Read the model definition and answer for the solid it produces. Units are mm, in the model's axes. A direction names the side the tool comes from. Coordinates: 2 decimals unless noted, no trailing zeros. Write each loop counter-clockwise with the first axis right and the second up, starting at its lowest first coordinate (ties: lowest second). Pieces come first, ordered by that corner, then holes. Notation, with made-up numbers: (11, 13) -> (48, 13) arc R35 ccw to (48, 51) -> close; hole circle Ø11 at (6, 52.25). An arc over 180 degrees is marked (long way). Answer in a Markdown table with one row per item. Add a question column.
Item 1: Section C-C on y = -12 is taken. Write down the section's boundary in (x, z), then the cut area to 3 significant figures.
Item 2: Section D-D on z = -22.5 is taken. Write down the section's boundary in (x, y).
Item 3: Given pin 1 Ø2.5 at (y, z) = (0, 22.5) entering from -X; pin 2 Ø2 at (x, y) = (-5, -8) entering from -Z; pin 3 Ø2 at (x, y) = (-5.5, -0.5) entering from +Z; pin 4 Ø4 at (y, z) = (2.5, 8) entering from -X, each flat-ended and moving along its own axis, determine where each tip first touches the part or whether it passes through.
Item 4: Section A-A on x = -2 is taken. Write down the section's boundary in (y, z), then the cut area to 3 significant figures.
Item 5: For a pull along X with two mould halves and no side action, classify faces 1 (the face through (4.3, 1.26, -16.62)), 2 (the face through (-3, -9, -12)), 3 (the face through (-4.285, 3.177, -8.031)), 4 (the face through (-5, -7, -8.332)) as +X half, -X half, draft (parallel to the pull), parting line (faces both ways), or undercut.
Item 6: Section B-B on y = -4.5 is taken. Write down the section's boundary in (x, z).
Item 7: Which of the six approach directions +Z, -Z, +X, -X, +Y, -Y give full straight-line access (tool end or side, diameter ignored) to faces 5 (the face through (0.056, -1.757, 11.526)), 6 (the face through (4.972, -11.934, -10.833)), 7 (the face through (-4, 2, 9)), 8 (the face through (-4, 1, -21)), 9 (the face through (3, -9, -12))?
Item 8: Straight lines are drawn through the part: line 1 (X direction, y = -5, z = -11.5); line 2 (Z direction, x = -3.9, y = -12); line 3 (Z direction, x = 5, y = -9.25). For each, find the intervals that lie inside material, in ascending order. Write a range as from..to.
```python
from build123d import *

# Parameters (mm, degrees)
CROQUIS1_R                          = 1.5
SALIENTE_EXTRUIR1_DEPTH             = 4
SALIENTE_EXTRUIR2_REACH             = 30.175
CROQUIS3_W                          = 3
CROQUIS3_H                          = 8
SALIENTE_EXTRUIR2_DIRECTION_2_REACH = 30.175
CROQUIS4_W                          = 14
CROQUIS4_H                          = 8
SALIENTE_EXTRUIR3_DEPTH             = 16
CORTAR_EXTRUIR2_REACH               = 38.892
CROQUIS7_W                          = 6
CROQUIS7_H                          = 8
REDONDEO1_R                         = 1
CORTAR_EXTRUIR1_DEPTH               = 32.737202145
CORTAR_EXTRUIR1_DEPTH_BACK          = 32.737202145
CROQUIS6_R                          = 1.5


with BuildPart() as part:
    # Croquis1 → Saliente-Extruir1 (new, symmetric)
    with BuildSketch(Plane(origin=(0, 0, 0), x_dir=(0, 0, -1), z_dir=(1, 0, 0))):
        with BuildLine():
            Line((-23.331646763, 3.912590403), (-1.663293527, 8.518341064))
            ThreePointArc((-1.663293527, 8.518341064), (0, 8.693160258), (1.663293527, 8.518341064))
            Line((1.663293527, 8.518341064), (23.331646763, 3.912590403))
            ThreePointArc((23.331646763, 3.912590403), (26.412590403, -0.831646763), (21.668353237, -3.912590403))
            Line((21.668353237, -3.912590403), (1.663293527, 0.339616305))
            ThreePointArc((1.663293527, 0.339616305), (0, 0.514435499), (-1.663293527, 0.339616305))
            Line((-1.663293527, 0.339616305), (-21.668353237, -3.912590403))
            ThreePointArc((-21.668353237, -3.912590403), (-26.412590403, -0.831646763), (-23.331646763, 3.912590403))
        make_face()
        with Locations((-22.5, 0)):
            Circle(CROQUIS1_R, mode=Mode.SUBTRACT)
        with Locations(Location((22.5, 0, 0), (0, 0, 180))):
            Circle(CROQUIS1_R, mode=Mode.SUBTRACT)
    extrude(amount=SALIENTE_EXTRUIR1_DEPTH, both=True)

    # Saliente-Extruir2: up to this plane
    saliente_extruir2_end = Plane(origin=(4, 0.339616305, -1.663293527), z_dir=(0, 0.9781476007338056, -0.20791169081776))
    # Croquis3 → Saliente-Extruir2 (add, up to the surface)
    with BuildSketch(Plane(origin=(0, 0, 0), x_dir=(1, 0, 0), z_dir=(0, 1, 0)), mode=Mode.PRIVATE) as saliente_extruir2_sk1:
        with Locations((-5.5, 12.331646763)):
            Rectangle(CROQUIS3_W, CROQUIS3_H)
    saliente_extruir2_tool1 = split(extrude(saliente_extruir2_sk1.sketch, amount=-SALIENTE_EXTRUIR2_REACH, mode=Mode.PRIVATE), bisect_by=saliente_extruir2_end, keep=Keep.BOTH, mode=Mode.PRIVATE)
    add(saliente_extruir2_tool1.solids().sort_by_distance((-5.5, 0, -12.331647))[0])
    # Croquis3 → Saliente-Extruir2 (add, up to the surface)
    with BuildSketch(Plane(origin=(0, 0, 0), x_dir=(1, 0, 0), z_dir=(0, 1, 0)), mode=Mode.PRIVATE) as saliente_extruir2_sk2:
        with Locations((5.5, 12.331646763)):
            Rectangle(CROQUIS3_W, CROQUIS3_H)
    saliente_extruir2_tool2 = split(extrude(saliente_extruir2_sk2.sketch, amount=-SALIENTE_EXTRUIR2_REACH, mode=Mode.PRIVATE), bisect_by=saliente_extruir2_end, keep=Keep.BOTH, mode=Mode.PRIVATE)
    add(saliente_extruir2_tool2.solids().sort_by_distance((5.5, 0, -12.331647))[0])

    # Saliente-Extruir2 direction 2: up to this plane
    saliente_extruir2_direction_2_end = Plane(origin=(4, 8.518341064, -1.663293527), z_dir=(0, -0.9781476007338056, 0.20791169081776004))
    # Croquis3 → Saliente-Extruir2 direction 2 (add, up to the surface)
    with BuildSketch(Plane(origin=(0, 0, 0), x_dir=(1, 0, 0), z_dir=(0, 1, 0)), mode=Mode.PRIVATE) as saliente_extruir2_direction_2_sk1:
        with Locations((-5.5, 12.331646763)):
            Rectangle(CROQUIS3_W, CROQUIS3_H)
    saliente_extruir2_direction_2_tool1 = split(extrude(saliente_extruir2_direction_2_sk1.sketch, amount=SALIENTE_EXTRUIR2_DIRECTION_2_REACH, mode=Mode.PRIVATE), bisect_by=saliente_extruir2_direction_2_end, keep=Keep.BOTH, mode=Mode.PRIVATE)
    add(saliente_extruir2_direction_2_tool1.solids().sort_by_distance((-5.5, 0, -12.331647))[0])
    # Croquis3 → Saliente-Extruir2 direction 2 (add, up to the surface)
    with BuildSketch(Plane(origin=(0, 0, 0), x_dir=(1, 0, 0), z_dir=(0, 1, 0)), mode=Mode.PRIVATE) as saliente_extruir2_direction_2_sk2:
        with Locations((5.5, 12.331646763)):
            Rectangle(CROQUIS3_W, CROQUIS3_H)
    saliente_extruir2_direction_2_tool2 = split(extrude(saliente_extruir2_direction_2_sk2.sketch, amount=SALIENTE_EXTRUIR2_DIRECTION_2_REACH, mode=Mode.PRIVATE), bisect_by=saliente_extruir2_direction_2_end, keep=Keep.BOTH, mode=Mode.PRIVATE)
    add(saliente_extruir2_direction_2_tool2.solids().sort_by_distance((5.5, 0, -12.331647))[0])

    # Croquis4 → Saliente-Extruir3 (add)
    with BuildSketch(Plane.XZ):
        with Locations((0, -12.331646763)):
            Rectangle(CROQUIS4_W, CROQUIS4_H)
    extrude(amount=SALIENTE_EXTRUIR3_DEPTH)

    # Cortar-Extruir2: up to this plane
    cortar_extruir2_end = Plane(origin=(4, 0.339616305, -1.663293527), z_dir=(0, 0.9781476007338056, -0.20791169081776))
    # Croquis7 → Cortar-Extruir2 (cut, up to the surface)
    with BuildSketch(Plane.XZ.offset(16), mode=Mode.PRIVATE) as cortar_extruir2_sk1:
        with Locations((0, -12.331646763)):
            Rectangle(CROQUIS7_W, CROQUIS7_H)
    cortar_extruir2_tool1 = split(extrude(cortar_extruir2_sk1.sketch, amount=-CORTAR_EXTRUIR2_REACH, mode=Mode.PRIVATE), bisect_by=cortar_extruir2_end, keep=Keep.BOTH, mode=Mode.PRIVATE)
    add(cortar_extruir2_tool1.solids().sort_by_distance((0, -16, -12.331647))[0], mode=Mode.SUBTRACT)

    # Redondeo1
    redondeo1_edges = [part.edges().sort_by_distance(p)[0] for p in [
        (4, 3.011576449, -8.331646763),
        (4, 1.311123955, -16.331646763),
        (-4, 3.011576449, -8.331646763),
        (-4, 1.311123955, -16.331646763),
        (3, -9.389119212, -16.331646763),
        (-3, -9.389119212, -16.331646763),
        (-3, -8.538892965, -8.331646763),
        (3, -8.538892965, -8.331646763),
        (7, -4.449530586, -8.331646763),
        (7, -5.299756833, -16.331646763),
        (-7, -5.299756833, -16.331646763),
        (-7, -4.449530586, -8.331646763),
    ]]
    fillet(redondeo1_edges, radius=REDONDEO1_R - 0.0001)  # a hair under: the kernel refuses the full size

    # Croquis6 → Cortar-Extruir1 (cut, two sides: drawn at the far end of the back side and taken through both)
    with BuildSketch(Plane(origin=(0, 0, 0), x_dir=(0, 0, -1), z_dir=(1, 0, 0)).offset(-CORTAR_EXTRUIR1_DEPTH_BACK)):
        with Locations((12.331646763, -12)):
            Circle(CROQUIS6_R)
    extrude(amount=CORTAR_EXTRUIR1_DEPTH + CORTAR_EXTRUIR1_DEPTH_BACK, mode=Mode.SUBTRACT)


solid = part.part
```
Results below:
| question | item | result |
|---|---|---|
| 1 | outline | (-7, -15.33) arc R1 ccw to (-6, -16.33) -> (-4, -16.33) arc R1 ccw to (-3, -15.33) -> (-3, -13.83) -> (-7, -13.83) -> close; (-7, -10.83) -> (-3, -10.83) -> (-3, -9.33) arc R1 ccw to (-4, -8.33) -> (-6, -8.33) arc R1 ccw to (-7, -9.33) -> close; (3, -15.33) arc R1 ccw to (4, -16.33) -> (6, -16.33) arc R1 ccw to (7, -15.33) -> (7, -13.83) -> (3, -13.83) -> close; (3, -10.83) -> (7, -10.83) -> (7, -9.33) arc R1 ccw to (6, -8.33) -> (4, -8.33) arc R1 ccw to (3, -9.33) -> close |
| 1 | area | 38.3 mm2 |
| 2 | outline | (-4, -4) -> (4, -4) -> (4, -1.5) -> (-4, -1.5) -> close; (-4, 1.5) -> (4, 1.5) -> (4, 4.09) -> (-4, 4.09) -> close |
| 3 | pin 1 | passes through |
| 3 | pin 2 | stops at z = -16.33 |
| 3 | pin 3 | stops at z = -8.2 |
| 3 | pin 4 | stops at x = -4 |
| 4 | outline | (-3.91, -21.67) arc R4 ccw to (3.91, -23.33) -> (8.52, -1.66) arc R8 ccw to (8.52, 1.66) -> (3.91, 23.33) arc R4 ccw to (-3.91, 21.67) -> (0.34, 1.66) arc R8 cw to (0.34, -1.66) -> close; hole circle Ø3 at (0, -22.5); hole circle Ø3 at (0, 22.5) |
| 4 | area | 404 mm2 |
| 5 | face 1 | +X half |
| 5 | face 2 | undercut |
| 5 | face 3 | -X half |
| 5 | face 4 | draft |
| 6 | outline | (-7, -15.33) arc R1 ccw to (-6, -16.33) -> (-4, -16.33) arc R1 ccw to (-3, -15.33) -> (-3, -9.33) arc R1 ccw to (-4, -8.33) -> (-6, -8.33) arc R1 ccw to (-7, -9.33) -> close; (3, -15.33) arc R1 ccw to (4, -16.33) -> (6, -16.33) arc R1 ccw to (7, -15.33) -> (7, -9.33) arc R1 ccw to (6, -8.33) -> (4, -8.33) arc R1 ccw to (3, -9.33) -> close |
| 7 | face 5 | +X, -X, -Y |
| 7 | face 6 | +X, -X |
| 7 | face 7 | +Z, -X, +Y, -Y |
| 7 | face 8 | -Z, -X, +Y, -Y |
| 7 | face 9 | -Y |
| 8 | line 1 | x = -7..-3, 3..7 |
| 8 | line 2 | z = -16.33..-13.83, -10.83..-8.34 |
| 8 | line 3 | z = -16.33..-8.33 |
